Geometry check sheet. Reference: drawing and pictorial views, mm from the part's lowest x, y, z. A direction names the side the tool comes from. Coordinates: 2 decimals unless noted, no trailing zeros. Order: outer loops, then holes, each group sorted by start corner. A loop starts at its lowest first (then second) coordinate and runs counter-clockwise, first axis right, second up. Notation, with made-up numbers: M -39.75,32 L -29.75,32 A27 cw -29.75,71 Z; hole C -22,-6.5 d5. An arc over 180 degrees is marked long. Return JSON: item names as keys, results as strings.
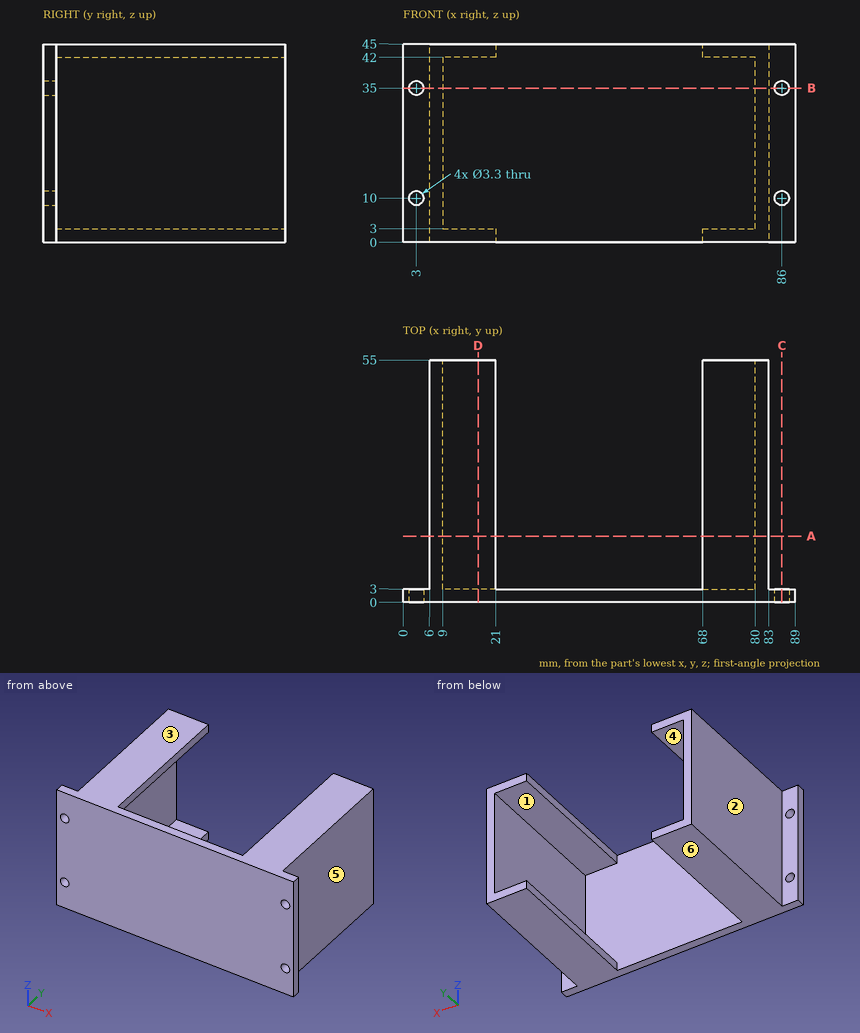
Q1. Cross-section at A-A, the plane y = 15. Record the boundary of the cut face in (x, z), and give its area (3 significant figures).
Values:
{"outline": "M 6,0 L 21,0 L 21,3 L 9,3 L 9,42 L 21,42 L 21,45 L 6,45 Z; M 68,0 L 83,0 L 83,45 L 68,45 L 68,42 L 80,42 L 80,3 L 68,3 Z", "area": "414 mm^2"}
Q2. Cross-section at B-B, the plane z = 35. Record the boundary of the cut face in (x, y), and give its area (3 significant figures).
Values:
{"outline": "M 0,0 L 1.35,0 L 1.35,3 L 0,3 Z; M 4.65,0 L 84.35,0 L 84.35,3 L 83,3 L 83,55 L 80,55 L 80,3 L 9,3 L 9,55 L 6,55 L 6,3 L 4.65,3 Z; M 87.65,0 L 89,0 L 89,3 L 87.65,3 Z", "area": "559 mm^2"}
Q3. Cross-section at C-C, the plane x = 86. Record the boundary of the cut face in (y, z), and give its area (3 significant figures).
Values:
{"outline": "M 0,0 L 3,0 L 3,8.35 L 0,8.35 Z; M 0,11.65 L 3,11.65 L 3,33.35 L 0,33.35 Z; M 0,36.65 L 3,36.65 L 3,45 L 0,45 Z", "area": "115 mm^2"}
Q4. Material ranges on line 1 along X through (y, z) = (1.1, 35); line 2 along Z through (x, y) = (3, 1.55); line 3 along X through (y, z) = (27, 41.5), recorded low to high.
Values:
{"line 1": "0 to 1.35, 4.65 to 84.35, 87.65 to 89", "line 2": "0 to 8.35, 11.65 to 33.35, 36.65 to 45", "line 3": "6 to 9, 80 to 83"}
Q5. Tool access check on the marked faces 1, 2 and 3. Record the directions out of +Z, -Z, +X, -X, +Y, -Y that give a thin tool (end or side, any length) a straight path to the whole face; none if there is none.
Values:
{"face 1": "+Y", "face 2": "+Z, -Z, -X, +Y", "face 3": "+Z, +X, -X, +Y, -Y"}
Q6. Go/stop test with flat-tipped pins: pin 1 (5.5 mm diameter, centred on x = 86, z = 10, fed in from +Y); pin 2 (2.5 mm diameter, centred on y = 27, z = 2, fed in from +X); pin 3 (22.5 mm diameter, centred on y = 17, z = 18, fed in from -X); pin 4 (1.5 mm diameter, centred on x = 13.5, z = 12.5, fed in from -Y). Record where each tip stops, or that it passes through.
Values:
{"pin 1": "y = 3", "pin 2": "x = 83", "pin 3": "x = 6", "pin 4": "y = 0"}
Q7. Draft check along X on the marked faces 4, 5 and 6. Enter one of: pulls with the +X half, pulls with the -X half, needs draft (parallel to the pull), parting line crosses it, or undercut.
Values:
{"face 4": "undercut", "face 5": "pulls with the +X half", "face 6": "needs draft"}
Q8. Cross-section at D-D, the plane x = 17. Record the boundary of the cut face in (y, z), and give its area (3 significant figures).
Values:
{"outline": "M 0,0 L 55,0 L 55,3 L 3,3 L 3,42 L 55,42 L 55,45 L 0,45 Z", "area": "447 mm^2"}
